For this review, take the finished solid that the model builds, in its own axes (mm). A direction names the side the tool comes from. Round coordinates to 2 decimals unless told otherwise and drop trailing zeros. Order: outer loops, then holes, each group sorted by start corner. A loop starts at its lowest first (then second) coordinate and runs counter-clockwise, first axis right, second up. Notation, with made-up numbers: (-8.5, 61) -> (8.5, 61) arc R16 ccw to (8.5, 83) -> close; hole circle Ø11 at (35, 17). An arc over 180 degrees is marked (long way). Use a Markdown table: item, result. Add a question column.
1) Consider section A-A (y = -45.5). State the section outline as (x, z) points, plus the area to 3 significant figures.
2) Consider section B-B (z = 21.5). State the section outline as (x, y) points.
3) Wall thickness on line 1 along Z through (x, y) = (1, -45); line 2 along Y through (x, z) = (1.6, 21.5); line 3 along Y through (x, z) = (3.8, 21.5): over which ranges is each line inside the solid? List them lowest first. Write a range as [from, to].
4) Consider section C-C (x = 30.5). State the section outline as (y, z) points, plus the area to 3 significant figures.
5) Clearance check with flat-ended pins moving along their axes: P1, Ø2, axis at y = 45.5, z = 9.5, coming from the -X side; P2, Ø4.5, axis at y = 44.5, z = 12.5, coming from the +X side; P3, Ø12, axis at x = 4.5, y = 2, coming from the +Z side; P4, Ø6, axis at x = 12.5, z = 14, coming from the +Y side. State where each tip first meets the part, or that it passes through.
6) Consider section D-D (y = 0). State the section outline as (x, z) points, plus the area to 3 significant figures.
7) Machinability: for faces 4 (the face through (12, 0, 7)), 5 (the face through (4, 0, 10)), 6 (the face through (5, 45, 15)), which of the approach directions +Z, -Z, +X, -X, +Y, -Y give a long, thin tool a straight path to every point of the face, cutting with its end or side? Answer none if there is none.
8) Draft analysis for pull direction Y (two halves, no side actions). For faces 1 (the face through (3, -51, 30)), 2 (the face through (32.99, -0.73, 17.82)), 3 (the face through (5, -45, 15)), state which applies: pulls with the +Y half, pulls with the -Y half, needs draft (parallel to the pull), parting line crosses it, or undercut.
```python
from build123d import *

# Parameters (mm, degrees)
SALIENTE_EXTRUIR1_DEPTH = 5
SALIENTE_EXTRUIR2_DEPTH = 26
SALIENTE_EXTRUIR3_DEPTH = 5
REDONDEO1_R             = 1
SALIENTE_EXTRUIR4_DEPTH = 26
REDONDEO2_R             = 5
CROQUIS5_R              = 1.25
CORTAR_EXTRUIR1_DEPTH   = 5


with BuildPart() as part:
    # Croquis1 → Saliente-Extruir1 (new body)
    with BuildSketch(Plane.XY):
        with BuildLine():
            Line((0, -38), (0, 38))
            Line((0, 38), (0, 53))
            Line((0, 53), (5, 53))
            Line((5, 53), (5, 37.669616404))
            ThreePointArc((5, 37.669616404), (38, 0), (5, -37.669616404))
            Line((5, -37.669616404), (5, -53))
            Line((5, -53), (0, -53))
            Line((0, -53), (0, -38))
        make_face()
    extrude(amount=SALIENTE_EXTRUIR1_DEPTH)

    # Croquis2 → Saliente-Extruir2 (add)
    with BuildSketch(Plane.XY.offset(5)):
        with BuildLine():
            Line((0, -38), (0, -33))
            ThreePointArc((0, -33), (33, 0), (0, 33))
            Line((0, 33), (0, 38))
            ThreePointArc((0, 38), (38, 0), (0, -38))
        make_face()
    extrude(amount=SALIENTE_EXTRUIR2_DEPTH)

    # Croquis3 → Saliente-Extruir3 (add)
    with BuildSketch(Plane.XY.offset(5)):
        with BuildLine():
            Line((0, 12), (0, -12))
            ThreePointArc((0, -12), (12, 0), (0, 12))
        make_face()
    extrude(amount=SALIENTE_EXTRUIR3_DEPTH)

    # Redondeo1
    redondeo1_edges = [part.edges().sort_by_distance(p)[0] for p in [
        (12, 0, 10),
    ]]
    fillet(redondeo1_edges, radius=REDONDEO1_R)

    # Croquis4 → Saliente-Extruir4 (add)
    with BuildSketch(Plane.XY.offset(5)):
        with BuildLine():
            Line((0, -38), (0, -53))
            Line((0, -53), (5, -53))
            Line((5, -53), (5, -37.669616404))
            ThreePointArc((5, -37.669616404), (2.505451722, -37.917314141), (0, -38))
        make_face()
        with BuildLine():
            Line((5, 37.669616404), (5, 53))
            Line((5, 53), (0, 53))
            Line((0, 53), (0, 38))
            ThreePointArc((0, 38), (2.505451722, 37.917314141), (5, 37.669616404))
        make_face()
    extrude(amount=SALIENTE_EXTRUIR4_DEPTH)

    # Redondeo2
    redondeo2_edges = [part.edges().sort_by_distance(p)[0] for p in [
        (2.5, 53, 0),
        (2.5, -53, 31),
        (2.5, 53, 31),
        (2.5, -53, 0),
    ]]
    fillet(redondeo2_edges, radius=REDONDEO2_R)

    # Croquis5 → Cortar-Extruir1 (cut)
    with BuildSketch(Plane.ZY):
        with Locations((9.5, 45.5)):
            Circle(CROQUIS5_R)
        with Locations((21.5, 45.5)):
            Circle(CROQUIS5_R)
        with Locations((21.5, -45.5)):
            Circle(CROQUIS5_R)
        with Locations((9.5, -45.5)):
            Circle(CROQUIS5_R)
    extrude(amount=-CORTAR_EXTRUIR1_DEPTH, mode=Mode.SUBTRACT)


solid = part.part
```
Results list:
| question | item | result |
|---|---|---|
| 1 | outline | (0, 0) -> (5, 0) -> (5, 8.25) -> (0, 8.25) -> close; (0, 10.75) -> (5, 10.75) -> (5, 20.25) -> (0, 20.25) -> close; (0, 22.75) -> (5, 22.75) -> (5, 31) -> (0, 31) -> close |
| 1 | area | 130 mm2 |
| 2 | outline | (0, -53) -> (5, -53) -> (5, -46.75) -> (0, -46.75) -> close; (0, -44.25) -> (5, -44.25) -> (5, -37.67) arc R38 ccw to (5, 37.67) -> (5, 44.25) -> (0, 44.25) -> (0, 33) arc R33 cw to (0, -33) -> close; (0, 46.75) -> (5, 46.75) -> (5, 53) -> (0, 53) -> close |
| 3 | line 1 | [0, 8.35], [10.65, 20.35], [22.65, 31] |
| 3 | line 2 | [-53, -46.75], [-44.25, -32.96], [32.96, 44.25], [46.75, 53] |
| 3 | line 3 | [-53, -46.75], [-44.25, -32.78], [32.78, 44.25], [46.75, 53] |
| 4 | outline | (-22.67, 0) -> (22.67, 0) -> (22.67, 31) -> (12.6, 31) -> (12.6, 5) -> (-12.6, 5) -> (-12.6, 31) -> (-22.67, 31) -> close |
| 4 | area | 750 mm2 |
| 5 | P1 | through |
| 5 | P2 | x = 5 |
| 5 | P3 | z = 10 |
| 5 | P4 | y = 36.79 |
| 6 | outline | (0, 0) -> (38, 0) -> (38, 31) -> (33, 31) -> (33, 5) -> (12, 5) -> (12, 9) arc R1 ccw to (11, 10) -> (0, 10) -> close |
| 6 | area | 380 mm2 |
| 7 | face 4 | +Z |
| 7 | face 5 | +Z, -X |
| 7 | face 6 | +Z, -Z, +X, +Y |
| 8 | face 1 | pulls with the -Y half |
| 8 | face 2 | undercut |
| 8 | face 3 | needs draft |
